Design review of the part built by this model. Coordinates are the model's own, in mm. A direction names the side the tool comes from. Coordinates: 2 decimals unless noted, no trailing zeros. Order: outer loops, then holes, each group sorted by start corner. A loop starts at its lowest first (then second) coordinate and runs counter-clockwise, first axis right, second up. Notation, with made-up numbers: (10.25, -3) -> (42.25, -3) arc R8 cw to (42.25, 11) -> close; hole circle Ø8 at (-18, -2.5). An arc over 180 degrees is marked (long way). Use a Markdown table: item, result. Add a question column.
Q1. Wall thickness on probe 1 along Z at (x, y) = (-2.45, -16.5); probe 2 along Y at (x, z) = (-5, 18.25); probe 3 along Y at (x, z) = (-13.8, 3): over which ranges is each line inside the solid? List them lowest first.
Q2. Machinability: for faces 1 (the face through (-1.97, -16.57, 1.35)), 2 (the face through (-6, -33, 11)), 3 (the face through (-7, -29, 11)), which of the approach directions +Z, -Z, +X, -X, +Y, -Y give a long, thin tool a straight path to every point of the face, cutting with its end or side? Answer none if there is none.
Q3. The part is to be moulded in two halves that separate along Y. For faces 4 (the face through (-6, 0, 11)), 5 (the face through (-12.72, -16.57, 1.35)), 6 (the face through (0, -16, 13)), say which applies: pulls with the +Y half, pulls with the -Y half, needs draft (parallel to the pull), parting line crosses it, or undercut.
Q4. Insertion check: pin 1 (2 mm diameter, centred on y = -16.5, z = 3, fed in from -X); pin 2 (6.5 mm diameter, centred on y = -15, z = 7, fed in from -X). Each pin has a flat end and moves straight along its axis. Give the tip position at first contact, or say it passes through.
Q5. Add section C-C (z = 4). State the section outline as (x, y) points.
Q6. Add section D-D (y = -16.5). State the section outline as (x, z) points, then the cut area to 3 significant figures.
Q7. Add section B-B (x = -8.5). State the section outline as (y, z) points, then the cut area to 3 significant figures.
Q8. Add section A-A (y = -28). State the section outline as (x, z) points.
from build123d import *

# Parameters (mm, degrees)
PAD_DEPTH       = 33
SKETCH001_W     = 6.5
SKETCH001_H     = 25
POCKET_DEPTH    = 30
SKETCH002_R     = 1.65
POCKET001_DEPTH = 15


with BuildPart() as part:
    # Sketch → Pad (new body)
    with BuildSketch(Plane.XZ):
        Polygon((-15.379194, 0), (0, 0), (0, 22), (-11.5, 22), align=None)
    extrude(amount=PAD_DEPTH)

    # Sketch001 (on Face3 of Pad) → Pocket (cut)
    with BuildSketch(Plane(origin=(0, 0, 22), x_dir=(-1, 0, 0), z_dir=(0, 0, 1))):
        with Locations((7.25, 16.5)):
            Rectangle(SKETCH001_W, SKETCH001_H)
    extrude(amount=-POCKET_DEPTH, mode=Mode.SUBTRACT)

    # Sketch002 (on Face5 of Pocket) → Pocket001 (cut)
    with BuildSketch(Plane(origin=(0, 0, 0), x_dir=(0, 0, 1), z_dir=(1, 0, 0))):
        with Locations((3, 16.5)):
            Circle(SKETCH002_R)
        with Locations((11, 16.5)):
            Circle(SKETCH002_R)
    extrude(amount=-POCKET001_DEPTH, mode=Mode.SUBTRACT)


solid = part.part
Established:
| question | item | result |
|---|---|---|
| 1 | probe 1 | 0 to 1.35, 4.65 to 9.35, 12.65 to 22 |
| 1 | probe 2 | -33 to -29, -4 to 0 |
| 1 | probe 3 | -33 to -18.15, -14.85 to 0 |
| 2 | face 1 | +X |
| 2 | face 2 | +Z, -Z, +X, -X, -Y |
| 2 | face 3 | +Z, -Z |
| 3 | face 4 | pulls with the +Y half |
| 3 | face 5 | undercut |
| 3 | face 6 | needs draft |
| 4 | pin 1 | x = -15.03 |
| 4 | pin 2 | x = -14.72 |
| 5 | outline | (-14.67, -33) -> (0, -33) -> (0, -17.81) -> (-4, -17.81) -> (-4, -29) -> (-10.5, -29) -> (-10.5, -17.81) -> (-14.67, -17.81) -> close; (-14.67, -15.19) -> (-10.5, -15.19) -> (-10.5, -4) -> (-4, -4) -> (-4, -15.19) -> (0, -15.19) -> (0, 0) -> (-14.67, 0) -> close |
| 6 | outline | (-15.38, 0) -> (-10.5, 0) -> (-10.5, 1.35) -> (-15, 1.35) -> (-15, 2.15) -> close; (-14.56, 4.65) -> (-10.5, 4.65) -> (-10.5, 9.35) -> (-13.73, 9.35) -> close; (-13.15, 12.65) -> (-10.5, 12.65) -> (-10.5, 22) -> (-11.5, 22) -> close; (-4, 0) -> (0, 0) -> (0, 1.35) -> (-4, 1.35) -> close; (-4, 4.65) -> (0, 4.65) -> (0, 9.35) -> (-4, 9.35) -> close; (-4, 12.65) -> (0, 12.65) -> (0, 22) -> (-4, 22) -> close |
| 6 | area | 102 mm^2 |
| 7 | outline | (-33, 0) -> (-29, 0) -> (-29, 22) -> (-33, 22) -> close; (-4, 0) -> (0, 0) -> (0, 22) -> (-4, 22) -> close |
| 7 | area | 176 mm^2 |
| 8 | outline | (-15.38, 0) -> (-10.5, 0) -> (-10.5, 22) -> (-11.5, 22) -> close; (-4, 0) -> (0, 0) -> (0, 22) -> (-4, 22) -> close |
